Source: CAD feature listing. Evaluate the final solid. Frame: model axes, mm. Face numbers are marked on the shaded views. A direction names the side the tool comes from. Round coordinates to 2 decimals unless told otherwise and drop trailing zeros. Loops run counter-clockwise (first coordinate to the right, second up) from the corner with the lowest first, then second, coordinate; pieces in that order, holes last. Notation, with made-up numbers: (89.5, -35.5) - (112.5, -35.5) arc R22 cw to (112.5, -14.5) - close; hole circle Ø7 at (-6.5, 26.5). An arc over 180 degrees is marked (long way). Write item = value, one per line. Start each with the question number.
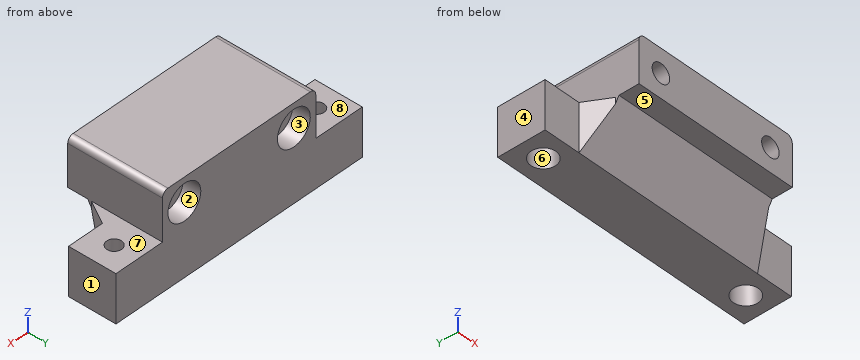
from build123d import *
from OCP.BRepFilletAPI import BRepFilletAPI_MakeChamfer

# Parameters (mm, degrees)
SKETCH_1_W           = 45
SKETCH_1_H           = 8
SKETCH_1_R           = 1.25
EXTRUDE_1_DEPTH      = 8
EXTRUDE_2_DEPTH      = 8
EXTRUDE_2_DEPTH_BACK = 8
SKETCH_2_W           = 28
SKETCH_2_H           = 8
SKETCH_2_R           = 1.6
SKETCH_4_R           = 3
CUT_EXTRUDE_2_DEPTH  = 3
FILLET_1_R           = 1
CHAMFER_1_SIZE2      = 8
CHAMFER_1_SIZE       = 4.618802154
CHAMFER_2_SIZE       = 4
CHAMFER_2_SIZE2      = 2.309401077
SKETCH_5_R           = 2.1
CUT_EXTRUDE_3_DEPTH  = 5


with BuildPart() as part:
    # ｽｹｯﾁ1 → ﾎﾞｽ - 押し出し1 (new body)
    with BuildSketch(Plane.XY):
        Rectangle(SKETCH_1_W, SKETCH_1_H)
        with Locations((-18.5, 0)):
            Circle(SKETCH_1_R, mode=Mode.SUBTRACT)
        with Locations(Location((18.5, 0, 0), (0, 0, 180))):
            Circle(SKETCH_1_R, mode=Mode.SUBTRACT)
    extrude(amount=EXTRUDE_1_DEPTH)

    # ｽｹｯﾁ2 → ﾎﾞｽ - 押し出し2 (add, two sides: drawn at the far end of the back side and taken through both)
    with BuildSketch(Plane.XZ.offset(4).offset(-EXTRUDE_2_DEPTH_BACK)):
        with Locations((0, 12)):
            Rectangle(SKETCH_2_W, SKETCH_2_H)
        with Locations(Location((-10, 12, 0), (0, 0, 270))):
            Circle(SKETCH_2_R, mode=Mode.SUBTRACT)
        with Locations(Location((10, 12, 0), (0, 0, 90))):
            Circle(SKETCH_2_R, mode=Mode.SUBTRACT)
    extrude(amount=EXTRUDE_2_DEPTH + EXTRUDE_2_DEPTH_BACK)

    # ｽｹｯﾁ4 → ｶｯﾄ - 押し出し2 (cut)
    with BuildSketch(Plane(origin=(0, 4, 0), x_dir=(1, 0, 0), z_dir=(0, 1, 0))):
        with Locations(Location((10, -12, 0), (0, 0, 270))):
            Circle(SKETCH_4_R)
        with Locations(Location((-10, -12, 0), (0, 0, 90))):
            Circle(SKETCH_4_R)
    extrude(amount=-CUT_EXTRUDE_2_DEPTH, mode=Mode.SUBTRACT)

    # ﾌｨﾚｯﾄ1
    fillet_1_edges = [part.edges().sort_by_distance(p)[0] for p in [
        (14, -4, 16),
        (-14, -4, 16),
    ]]
    fillet(fillet_1_edges, radius=FILLET_1_R)

    # 面取り1
    chamfer_1_edges = [part.edges().sort_by_distance(p)[0] for p in [
        (0, -4, 8),
    ]]
    chamfer_1_side = [part.faces().sort_by_distance(p)[0] for p in [
        (0, -4.092376043, 8),
    ]]
    chamfer(chamfer_1_edges, length=CHAMFER_1_SIZE - 0.0001, length2=CHAMFER_1_SIZE2 - 0.0001, reference=chamfer_1_side[0])  # a hair under: the kernel refuses the full size

    # 面取り2: one chamfer whose edges measure the first distance from different faces: ONE call of the kernel's chamfer builder (chamfer() names one face for all edges)
    chamfer_2_edges_1 = [part.edges().sort_by_distance(p)[0] for p in [
        (-14, -4, 4.00005),
    ]]
    chamfer_2_side_1 = [part.faces().sort_by_distance(p)[0] for p in [
        (-14, -4.217995396, 10.626834142),
    ]]
    chamfer_2_edges_2 = [part.edges().sort_by_distance(p)[0] for p in [
        (14, -4, 4.00005),
    ]]
    chamfer_2_side_2 = [part.faces().sort_by_distance(p)[0] for p in [
        (14, -4.217995396, 10.626834142),
    ]]
    chamfer_2 = BRepFilletAPI_MakeChamfer(part.part.solid().wrapped)
    for e in chamfer_2_edges_1:
        chamfer_2.Add(CHAMFER_2_SIZE, CHAMFER_2_SIZE2, e.wrapped, chamfer_2_side_1[0].wrapped)  # the first distance lies on this face
    for e in chamfer_2_edges_2:
        chamfer_2.Add(CHAMFER_2_SIZE, CHAMFER_2_SIZE2, e.wrapped, chamfer_2_side_2[0].wrapped)  # the first distance lies on this face
    add(Compound.cast(chamfer_2.Shape()), mode=Mode.REPLACE)

    # ｽｹｯﾁ5 → ｶｯﾄ - 押し出し3 (cut)
    with BuildSketch(Plane(origin=(0, 0, 0), x_dir=(-1, 0, 0), z_dir=(0, 0, -1))):
        with Locations((-18.5, 0)):
            Circle(SKETCH_5_R)
        with Locations((18.5, 0)):
            Circle(SKETCH_5_R)
    extrude(amount=-CUT_EXTRUDE_3_DEPTH, mode=Mode.SUBTRACT)


solid = part.part
(1) Cut plane A-A (y = 0). Output: boundary loops of the cut face in (x, z), and give its area (3 significant figures).
(2) Cut plane D-D (y = -9.5). Output: boundary loops of the cut face in (x, z).
(3) Cut plane B-B (x = -18.5). Output: boundary loops of the cut face in (y, z), and give its area (3 significant figures).
(4) Pin query (flat end, axial travel): P1, Ø2, axis at x = 18, y = 0.5, coming from the -Z side; P2, Ø2, axis at x = -18.5, y = 0, coming from the +Z side; P3, Ø4, axis at x = 18.5, y = 0, coming from the +Z side; P4, Ø9, axis at x = 3.5, z = 2.5, coming from the -Y side. Return the tip coordinate at first contact, or that it passes through.
(5) Access query for the marked faces 5, 6, 7 and 8. Directions: +Z, -Z, +X, -X, +Y, -Y. A direction counts if a zero-diameter tool reaches every point of the face in a straight line with its end or side. Return the directions, or none.
(6) Mould query, pull axis X, two halves, no side actions, for the marked faces 1, 2, 3 and 4. Classes: +X half, -X half, draft (parallel to the pull), parting line (faces both ways), or undercut.
(7) Cut plane C-C (z = 12). Output: boundary loops of the cut face in (x, y).
(8) Material intervals for line 1 along X through (y, z) = (2.3, 12); line 2 along Y through (x, z) = (18.5, 7.3); line 3 along X through (y, z) = (-4, 12), sorted ascending. Write a range as from..to.
Solution:
q1.outline = (-22.5, 0) - (-20.6, 0) - (-20.6, 5) - (-19.75, 5) - (-19.75, 8) - (-22.5, 8) - close; (-17.25, 5) - (-16.4, 5) - (-16.4, 0) - (16.4, 0) - (16.4, 5) - (17.25, 5) - (17.25, 8) - (14, 8) - (14, 15) arc R1 ccw to (13, 16) - (-13, 16) arc R1 ccw to (-14, 15) - (-14, 8) - (-17.25, 8) - close; (19.75, 5) - (20.6, 5) - (20.6, 0) - (22.5, 0) - (22.5, 8) - (19.75, 8) - close; hole circle Ø3.2 at (-10, 12); hole circle Ø3.2 at (10, 12)
q1.area = 510 mm^2
q2.outline = (-14, 8) - (14, 8) - (14, 15) arc R1 ccw to (13, 16) - (-13, 16) arc R1 ccw to (-14, 15) - close; hole circle Ø3.2 at (-10, 12); hole circle Ø3.2 at (10, 12)
q3.outline = (-4, 0) - (-2.1, 0) - (-2.1, 5) - (-1.25, 5) - (-1.25, 8) - (-4, 8) - close; (1.25, 5) - (2.1, 5) - (2.1, 0) - (4, 0) - (4, 8) - (1.25, 8) - close
q3.area = 35.5 mm^2
q4.P1 = 5
q4.P2 = through
q4.P3 = 8
q4.P4 = -8.04
q5.face_5 = -Z, +X, -X, -Y
q5.face_6 = -Z
q5.face_7 = +Z, +X, +Y, -Y
q5.face_8 = +Z, -X, +Y, -Y
q6.face_1 = +X half
q6.face_2 = undercut
q6.face_3 = undercut
q6.face_4 = -X half
q7.outline = (-14, -12) - (-11.6, -12) - (-11.6, 1) - (-13, 1) - (-13, 4) - (-14, 4) - close; (-8.4, -12) - (8.4, -12) - (8.4, 1) - (7, 1) - (7, 4) - (-7, 4) - (-7, 1) - (-8.4, 1) - close; (11.6, -12) - (14, -12) - (14, 4) - (13, 4) - (13, 1) - (11.6, 1) - close
q8.line_1 = -14..-13, -7..7, 13..14
q8.line_2 = -4..-1.25, 1.25..4
q8.line_3 = -14..-11.6, -8.4..8.4, 11.6..14
